Job drawing, mm, ordinate dimensions from the low corner. One solid piece. Give positions to 0.01 mm unless a question says otherwise; leave off trailing zeros. Order: outer loops, then holes, each group sorted by start corner. A loop starts at its lowest first (then second) coordinate and runs counter-clockwise, first axis right, second up.
Item 1: Two-plate mould, pull along Z, no slides. Class the marked faces 1, 2 and 3: released by +Z, released by -Z, zero draft, split by the parting line, or undercut.
Item 2: Wall check: L1, parallel to X at y = 6.5, z = 7.5; L2, parallel to Z at x = 5.5, y = 8; L3, parallel to Y at x = 13, z = 6.25. Give the ranges that are in metal, low to high.
Item 3: Flat gauge pins, fed straight in: P1, Ø4, axis at y = 6.5, z = 11, coming from the -X side; P2, Ø5, axis at x = 37, z = 10.5, coming from the -Y side; P3, Ø0.5, axis at x = 31, y = 6, coming from the +Z side; P4, Ø4, axis at x = 9.5, y = 3, coming from the +Z side. Where does each tip first touch, or does it go through?
Item 4: Band-saw the part on D-D on z = 10.5. Give the cut face in (x, y).
Item 5: Band-saw the part on B-B on z = 8. Count the separate pieces of the cut face and the enclosed holes in it, plus the area to 3 significant figures.
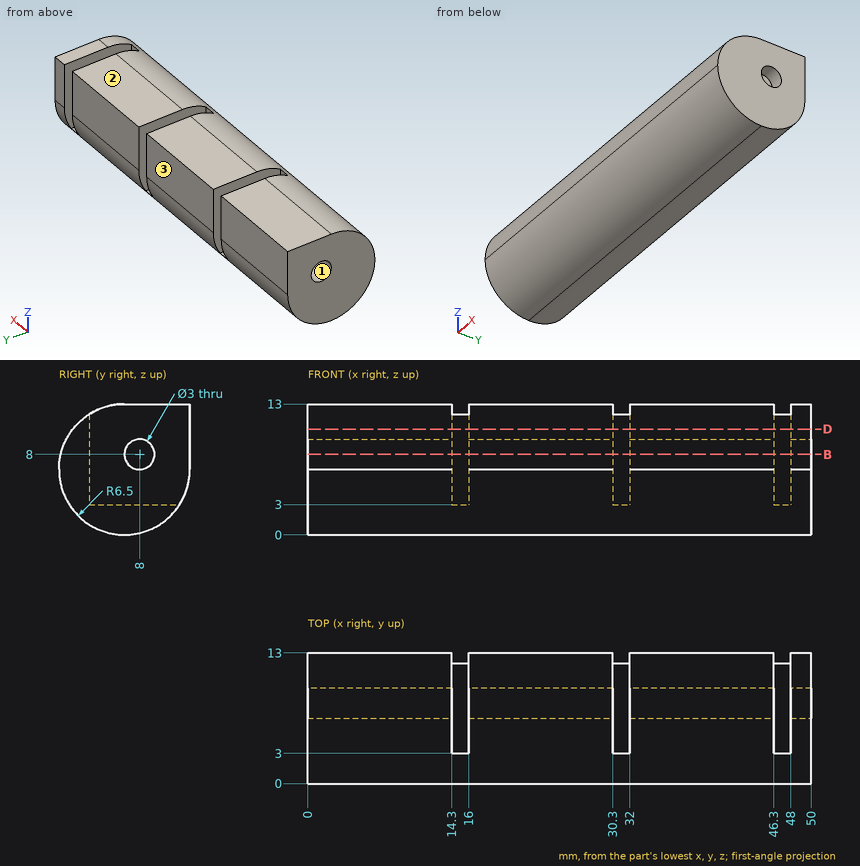
The answers:
1. face 1: undercut
1. face 2: released by +Z
1. face 3: zero draft
2. L1: x = 0 to 14.3, 16 to 30.3, 32 to 46.3, 48 to 50
2. L2: z = 0.18 to 6.5, 9.5 to 13
2. L3: y = 0 to 13
3. P1: stops at x = 0
3. P2: stops at y = 0.18
3. P3: stops at z = 3
3. P4: stops at z = 12.82
4. outline: (0, 1.38) - (50, 1.38) - (50, 13) - (48, 13) - (48, 3) - (46.3, 3) - (46.3, 13) - (32, 13) - (32, 3) - (30.3, 3) - (30.3, 13) - (16, 13) - (16, 3) - (14.3, 3) - (14.3, 13) - (0, 13) - close
5. separate pieces: 5
5. enclosed holes: 0
5. area: 456 mm2
